Build history of the part. All positions in model axes, mm. A direction names the side the tool comes from. Coordinates: 2 decimals unless noted, no trailing zeros. Order: outer loops, then holes, each group sorted by start corner. A loop starts at its lowest first (then second) coordinate and runs counter-clockwise, first axis right, second up. Notation, with made-up numbers: (-6.5, -7) -> (20.5, -7) arc R25 cw to (20.5, 24) -> close; hole circle Ø10 at (-34, 52.5). An arc over 180 degrees is marked (long way). Write each question's results on one line, items separated by ' | '.
from build123d import *

# Parameters (mm, degrees)
SKETCH_W        = 310
SKETCH_H        = 110
PAD_DEPTH       = 8
PAD001_DEPTH    = 110
POCKET_DEPTH    = 500
POCKET001_DEPTH = 500
SKETCH006_R     = 2.625
POCKET002_DEPTH = 500
SKETCH007_W     = 298
SKETCH007_H     = 8
POCKET003_DEPTH = 102
SKETCH009_W     = 300
SKETCH009_H     = 1.5
POCKET004_DEPTH = 110
SKETCH010_W     = 290
SKETCH010_H     = 10
POCKET005_DEPTH = 110
SKETCH011_R     = 2.1
POCKET006_DEPTH = 500


with BuildPart() as part:
    # Sketch → Pad (new body)
    with BuildSketch(Plane.XY):
        with Locations((155, 55)):
            Rectangle(SKETCH_W, SKETCH_H)
    extrude(amount=PAD_DEPTH)

    # Sketch001 (on Face6 of Pad) → Pad001 (join)
    with BuildSketch(Plane.XY.offset(8)):
        Polygon((0, 0), (0, 110), (310, 110), (310, 0), (305, 0), (305, 105), (5, 105), (5, 0), align=None)
    extrude(amount=PAD001_DEPTH)

    # Sketch004 (on Face9 of Pad001) → Pocket (cut)
    with BuildSketch(Plane(origin=(0, 0, 0), x_dir=(0, -1, 0), z_dir=(-1, 0, 0))):
        Polygon((-100, 118), (0, 118), (0, 8), align=None)
    extrude(amount=-POCKET_DEPTH, mode=Mode.SUBTRACT)

    # Sketch005 (on Face9 of Pocket) → Pocket001 (cut)
    with BuildSketch(Plane(origin=(0, 0, 0), x_dir=(0, -1, 0), z_dir=(-1, 0, 0))):
        Polygon((-100, 113), (-5, 8), (-105, 8), (-105, 113), align=None)
    extrude(amount=-POCKET001_DEPTH, mode=Mode.SUBTRACT)

    # Sketch006 (on Face1 of Pocket001) → Pocket002 (cut)
    with BuildSketch(Plane.XZ):
        with Locations((5, 4)):
            Circle(SKETCH006_R)
        with Locations((305, 4)):
            Circle(SKETCH006_R)
    extrude(amount=-POCKET002_DEPTH, mode=Mode.SUBTRACT)

    # Sketch007 (on Face1 of Pocket002) → Pocket003 (cut)
    with BuildSketch(Plane.XZ):
        with Locations((155, 4)):
            Rectangle(SKETCH007_W, SKETCH007_H)
    extrude(amount=-POCKET003_DEPTH, mode=Mode.SUBTRACT)

    # Sketch009 (on Face17 of Pocket003) → Pocket004 (cut)
    with BuildSketch(Plane.XY.offset(118)):
        with Locations((155, 107.25)):
            Rectangle(SKETCH009_W, SKETCH009_H)
    extrude(amount=-POCKET004_DEPTH, mode=Mode.SUBTRACT)

    # Sketch010 (on Face17 of Pocket004) → Pocket005 (cut)
    with BuildSketch(Plane.XY.offset(118)):
        with Locations((155, 107)):
            Rectangle(SKETCH010_W, SKETCH010_H)
    extrude(amount=-POCKET005_DEPTH, mode=Mode.SUBTRACT)

    # Sketch011 (on Face13 of Pocket005) → Pocket006 (cut)
    with BuildSketch(Plane.XZ.offset(-102)):
        with Locations((30, 4)):
            Circle(SKETCH011_R)
        with Locations((280, 4)):
            Circle(SKETCH011_R)
    extrude(amount=-POCKET006_DEPTH, mode=Mode.SUBTRACT)


solid = part.part
Item 1: Pull direction Y, two halves, no side cores. Call faces 1 (the flat face through (153, 102, 4)), 2 (the flat face through (310, 63, 6)), 3 (the flat face through (2.46, 53.16, 61.23)): released by +Y, released by -Y, zero draft, split by the parting line, or undercut.
Answer:
face 1: released by -Y | face 2: zero draft | face 3: undercut
Item 2: Slice it at B-B, the plane z = 87.5. List the corners of the cut face in (x, y), and give its area (3 significant figures).
Answer:
outline: (0, 72.27) -> (5, 72.27) -> (5, 76.93) -> (0, 76.93) -> close; (0, 105) -> (10, 105) -> (10, 106.5) -> (5, 106.5) -> (5, 108) -> (10, 108) -> (10, 110) -> (0, 110) -> close; (300, 105) -> (310, 105) -> (310, 110) -> (300, 110) -> (300, 108) -> (305, 108) -> (305, 106.5) -> (300, 106.5) -> close; (305, 72.27) -> (310, 72.27) -> (310, 76.93) -> (305, 76.93) -> close | area: 132 mm^2
Item 3: Drill centre lines: line 1 (X direction, y = 35, z = 4) (3 decimals); line 2 (Y direction, x = 116, z = 5); line 3 (X direction, y = 59, z = 71.5). Where is each one in solid material? Low to high. Write a range as from..to.
Answer:
line 1: x = 0..2.375, 307.625..310 | line 2: y = 102..110 | line 3: x = 0..5, 305..310
Item 4: Pin check, flat tips, straight feed: pin 1 (11 mm diameter, centred on x = 306, z = 39.5, fed in from -Y); pin 2 (4 mm diameter, centred on x = 5, z = 4, fed in from +Y); pin 3 (2.5 mm diameter, centred on x = 301.5, z = 55, fed in from -Y). Stop position of each tip, or through.
Answer:
pin 1: stops at y = 23.64 | pin 2: passes through | pin 3: stops at y = 105
Item 5: Slice it at C-C, the plane y = 14. List the corners of the cut face in (x, z) (3 decimals).
Answer:
outline: (0, 0) -> (6, 0) -> (6, 1.573) arc R2.625 cw (long way) to (6, 6.427) -> (6, 8) -> (0, 8) -> close; (0, 17.947) -> (5, 17.947) -> (5, 23.4) -> (0, 23.4) -> close; (304, 0) -> (310, 0) -> (310, 8) -> (304, 8) -> (304, 6.427) arc R2.625 cw (long way) to (304, 1.573) -> close; (305, 17.947) -> (310, 17.947) -> (310, 23.4) -> (305, 23.4) -> close
Item 6: Tool access for faces 4 (the flat face through (308, 0, 4)), 5 (the flat face through (307.46, 53.16, 61.23)), 6 (the flat face through (5, 53, 63)): list every direction of +Z, -Z, +X, -X, +Y, -Y with a clear straight run to the whole face (end or side of a thin tool).
Answer:
face 4: +Z, -Z, +X, -X, -Y | face 5: +X, -X | face 6: +Z, -Y
Item 7: Slice it at A-A, the plane y = 62. List the corners of the cut face in (x, z) (3 decimals).
Answer:
outline: (0, 0) -> (6, 0) -> (6, 1.573) arc R2.625 cw (long way) to (6, 6.427) -> (6, 8) -> (0, 8) -> close; (0, 71) -> (5, 71) -> (5, 76.2) -> (0, 76.2) -> close; (304, 0) -> (310, 0) -> (310, 8) -> (304, 8) -> (304, 6.427) arc R2.625 cw (long way) to (304, 1.573) -> close; (305, 71) -> (310, 71) -> (310, 76.2) -> (305, 76.2) -> close
Item 8: Slice it at D-D, the plane x = 164.5. List the corners of the cut face in (y, z).
Answer:
outline: (102, 0) -> (110, 0) -> (110, 8) -> (102, 8) -> close
